Work out the finished part from the listing and answer in its coordinate system (mm). A direction names the side the tool comes from. Coordinates: 2 decimals unless noted, no trailing zeros. Loops run counter-clockwise (first coordinate to the right, second up) from the corner with the lowest first, then second, coordinate; pieces in that order, holes last. Notation, with made-up numbers: (1.25, 5) -> (31.25, 5) arc R22 cw to (31.25, 15) -> close; hole circle Ø8 at (48.25, 15.25). An arc over 180 degrees is marked (long way). Use a Markdown table: item, result.
from build123d import *

# Parameters (mm, degrees)
F0_W     = 150
F0_H     = 100
F1_DEPTH = 25
F2_R     = 2.5
F3_DEPTH = 15
F4_R     = 2.5
F5_DEPTH = 15


with BuildPart() as f1:
    # F0 (on Front) → F1 (new body)
    with BuildSketch(Plane.XZ):
        Rectangle(F0_W, F0_H)
    extrude(amount=F1_DEPTH)

    # F2 (on face) → F3 (join)
    with BuildSketch(Plane.XZ.offset(25)):
        with Locations((-30, 0)):
            Circle(F2_R)
    extrude(amount=F3_DEPTH)

    # F4 (on face) → F5 (join)
    with BuildSketch(Plane.XZ.offset(25)):
        with Locations((-5, 0)):
            Circle(F4_R)
    extrude(amount=F5_DEPTH)


solid = f1.part
Q1. Section B-B on z = 0 is taken. Determine the outline of the cut face in (x, y).
Solved:
| item | result |
|---|---|
| outline | (-75, -25) -> (-32.5, -25) -> (-32.5, -40) -> (-27.5, -40) -> (-27.5, -25) -> (-7.5, -25) -> (-7.5, -40) -> (-2.5, -40) -> (-2.5, -25) -> (75, -25) -> (75, 0) -> (-75, 0) -> close |
Q2. Consider line 1 (Y direction, x = -51, z = -20.5); line 2 (Z direction, x = -29, y = -37). Determine where each line is inside the solid, lowest interval first. Write a range as [from, to].
Solved:
| item | result |
|---|---|
| line 1 | [-25, 0] |
| line 2 | [-2.29, 2.29] |
Q3. Section A-A on x = -30 is taken. Determine the outline of the cut face in (y, z).
Solved:
| item | result |
|---|---|
| outline | (-40, -2.5) -> (-25, -2.5) -> (-25, -50) -> (0, -50) -> (0, 50) -> (-25, 50) -> (-25, 2.5) -> (-40, 2.5) -> close |
Q4. Given pin 1 Ø12 at (x, z) = (-53.5, 27.5) entering from -Y, flat-ended and moving along its own axis, determine where the tip first touches the part or whether it passes through.
Solved:
| item | result |
|---|---|
| pin 1 | y = -25 |
Q5. For faces 1 (the cylindrical face through (-32.5, -32.4, 0.1)), 2 (the flat face through (-1, -12, 50)), determine the directions among +Z, -Z, +X, -X, +Y, -Y from which every point of the face is accessible in a straight line to the end or side of a thin tool.
Solved:
| item | result |
|---|---|
| face 1 | -Y |
| face 2 | +Z, +X, -X, +Y, -Y |
Q6. Section C-C on y = -34 is taken. Determine the outline of the cut face in (x, z), and give its area (3 significant figures).
Solved:
| item | result |
|---|---|
| outline | circle Ø5 at (-30, 0); circle Ø5 at (-5, 0) |
| area | 39.3 mm² |
Q7. Section D-D on z = -36.5 is taken. Determine the outline of the cut face in (x, y), and give its area (3 significant figures).
Solved:
| item | result |
|---|---|
| outline | (-75, -25) -> (75, -25) -> (75, 0) -> (-75, 0) -> close |
| area | 3,750 mm² |
Q8. Determine the mould class of faces 3 (the flat face through (-75, -12, -1)), 4 (the flat face through (-30, -40, 0)), 5 (the flat face through (75, -12, -1)), 6 (the cylindrical face through (-2.615, -32.395, 0.751)) for opening direction X: pulls with the +X half, pulls with the -X half, needs draft (parallel to the pull), parting line crosses it, or undercut.
Solved:
| item | result |
|---|---|
| face 3 | pulls with the -X half |
| face 4 | needs draft |
| face 5 | pulls with the +X half |
| face 6 | undercut |
